```python
from build123d import *

# Parameters (mm, degrees)
ESQUISSE1_W              = 137
ESQUISSE1_H              = 66
BOSS_EXTRU_2_DEPTH       = 15
ESQUISSE3_W              = 131
ESQUISSE3_H              = 60
ENL_V_MAT_EXTRU_1_DEPTH  = 10
ESQUISSE5_W              = 12
ESQUISSE5_H              = 12
ENL_V_MAT_EXTRU_2_DEPTH  = 10
ESQUISSE6_W              = 12
ESQUISSE6_H              = 12
ENL_V_MAT_EXTRU_3_DEPTH  = 10
ESQUISSE7_W              = 15
ESQUISSE7_H              = 3
ENL_V_MAT_EXTRU_4_DEPTH  = 10
ESQUISSE8_R              = 4.5
ENL_V_MAT_EXTRU_5_DEPTH  = 10
ESQUISSE10_W             = 3
ESQUISSE10_H             = 8
BOSS_EXTRU_3_DEPTH       = 4
ESQUISSE12_W             = 2
ESQUISSE12_H             = 6
ENL_V_MAT_EXTRU_6_DEPTH  = 4
ESQUISSE13_W             = 3
ESQUISSE13_H             = 8
BOSS_EXTRU_4_DEPTH       = 4
ESQUISSE14_W             = 2
ESQUISSE14_H             = 6
ENL_V_MAT_EXTRU_7_DEPTH  = 4
ESQUISSE16_W             = 3
ESQUISSE16_H             = 8
BOSS_EXTRU_5_DEPTH       = 4
ESQUISSE17_W             = 3
ESQUISSE17_H             = 8
BOSS_EXTRU_6_DEPTH       = 4
ESQUISSE19_W             = 2
ESQUISSE19_H             = 6
ENL_V_MAT_EXTRU_9_DEPTH  = 3
ESQUISSE20_W             = 2
ESQUISSE20_H             = 6
ENL_V_MAT_EXTRU_10_DEPTH = 3
ESQUISSE21_R             = 1.5
ENL_V_MAT_EXTRU_12_DEPTH = 21
ESQUISSE22_W             = 3
ESQUISSE22_H             = 8
ENL_V_MAT_EXTRU_13_DEPTH = 4
ESQUISSE23_W             = 3
ESQUISSE23_H             = 8
ENL_V_MAT_EXTRU_14_DEPTH = 4
ESQUISSE24_W             = 3
ESQUISSE24_H             = 8
ENL_V_MAT_EXTRU_15_DEPTH = 4
ESQUISSE25_W             = 3
ESQUISSE25_H             = 8
ENL_V_MAT_EXTRU_16_DEPTH = 4
ESQUISSE28_W             = 12
ESQUISSE28_H             = 12
BOSS_EXTRU_7_DEPTH       = 5
ESQUISSE30_W             = 9
ESQUISSE30_H             = 9
ENL_V_MAT_EXTRU_17_DEPTH = 2.5
ESQUISSE32_W             = 9
ESQUISSE32_H             = 9
ENL_V_MAT_EXTRU_18_DEPTH = 8.5
ESQUISSE33_W             = 16
ESQUISSE33_H             = 16
ENL_V_MAT_EXTRU_19_DEPTH = 3
ESQUISSE34_W             = 16
ESQUISSE34_H             = 16
ENL_V_MAT_EXTRU_20_DEPTH = 3
ESQUISSE35_W             = 9
ESQUISSE35_H             = 9
ENL_V_MAT_EXTRU_21_DEPTH = 3
ESQUISSE36_W             = 12
ESQUISSE36_H             = 12
BOSS_EXTRU_8_DEPTH       = 5
ESQUISSE37_R             = 2.5
ENL_V_MAT_EXTRU_22_DEPTH = 5
ESQUISSE39_W             = 3
ESQUISSE39_H             = 60
ENL_V_MAT_EXTRU_23_DEPTH = 10
ESQUISSE40_W             = 5
ESQUISSE40_H             = 66
BOSS_EXTRU_9_DEPTH       = 7
ESQUISSE41_W             = 3
ESQUISSE41_H             = 66
BOSS_EXTRU_10_DEPTH      = 10
ESQUISSE42_W             = 4
ESQUISSE42_H             = 3
BOSS_EXTRU_11_DEPTH      = 10
ESQUISSE43_W             = 4
ESQUISSE43_H             = 3
BOSS_EXTRU_12_DEPTH      = 10
ESQUISSE44_W             = 20
ESQUISSE44_H             = 8
ENL_V_MAT_EXTRU_24_DEPTH = 10
ESQUISSE46_W             = 138
ESQUISSE46_H             = 3
ENL_V_MAT_EXTRU_25_DEPTH = 10
ESQUISSE47_W             = 141
ESQUISSE47_H             = 5
BOSS_EXTRU_13_DEPTH      = 7
ESQUISSE48_W             = 141
ESQUISSE48_H             = 3.004636282
BOSS_EXTRU_14_DEPTH      = 10
ESQUISSE49_W             = 3
ESQUISSE49_H             = 3.995363718
BOSS_EXTRU_15_DEPTH      = 10
ESQUISSE50_W             = 3
ESQUISSE50_H             = 15
BOSS_EXTRU_16_DEPTH      = 7


with BuildPart() as part:
    # Esquisse1 → Boss.-Extru.2 (new body)
    with BuildSketch(Plane.XY):
        with Locations((68.5, 33)):
            Rectangle(ESQUISSE1_W, ESQUISSE1_H)
    extrude(amount=BOSS_EXTRU_2_DEPTH)

    # Esquisse3 → Enlèv. mat.-Extru.1 (cut)
    with BuildSketch(Plane.XY.offset(15)):
        with Locations((68.5, 33)):
            Rectangle(ESQUISSE3_W, ESQUISSE3_H)
    extrude(amount=-ENL_V_MAT_EXTRU_1_DEPTH, mode=Mode.SUBTRACT)

    # Esquisse5 → Enlèv. mat.-Extru.2 (cut)
    with BuildSketch(Plane(origin=(0, 0, 0), x_dir=(-1, 0, 0), z_dir=(0, 0, -1))):
        with Locations((-14.887820014, 52.506524993)):
            Rectangle(ESQUISSE5_W, ESQUISSE5_H)
    extrude(amount=-ENL_V_MAT_EXTRU_2_DEPTH, mode=Mode.SUBTRACT)

    # Esquisse6 → Enlèv. mat.-Extru.3 (cut)
    with BuildSketch(Plane(origin=(0, 0, 0), x_dir=(-1, 0, 0), z_dir=(0, 0, -1))):
        with Locations((-42.758546676, 52.506524993)):
            Rectangle(ESQUISSE6_W, ESQUISSE6_H)
    extrude(amount=-ENL_V_MAT_EXTRU_3_DEPTH, mode=Mode.SUBTRACT)

    # Esquisse7 → Enlèv. mat.-Extru.4 (cut)
    with BuildSketch(Plane(origin=(0, 0, 0), x_dir=(-1, 0, 0), z_dir=(0, 0, -1))):
        with Locations((-55.331883335, 4.5)):
            Rectangle(ESQUISSE7_W, ESQUISSE7_H)
    extrude(amount=-ENL_V_MAT_EXTRU_4_DEPTH, mode=Mode.SUBTRACT)

    # Esquisse8 → Enlèv. mat.-Extru.5 (cut)
    with BuildSketch(Plane(origin=(0, 0, 0), x_dir=(-1, 0, 0), z_dir=(0, 0, -1))):
        with Locations((-69.128546676, 52.506524993)):
            Circle(ESQUISSE8_R)
    extrude(amount=-ENL_V_MAT_EXTRU_5_DEPTH, mode=Mode.SUBTRACT)

    # Esquisse10 → Boss.-Extru.3 (add)
    with BuildSketch(Plane.XY.offset(5)):
        with Locations((7.387820014, 52.506524993)):
            Rectangle(ESQUISSE10_W, ESQUISSE10_H)
    extrude(amount=BOSS_EXTRU_3_DEPTH)

    # Esquisse12 → Enlèv. mat.-Extru.6 (cut)
    with BuildSketch(Plane(origin=(8.887820014, 0, 0), x_dir=(0, 0, -1), z_dir=(1, 0, 0))):
        with Locations((-7, 52.506524993)):
            Rectangle(ESQUISSE12_W, ESQUISSE12_H)
    extrude(amount=-ENL_V_MAT_EXTRU_6_DEPTH, mode=Mode.SUBTRACT)

    # Esquisse13 → Boss.-Extru.4 (add)
    with BuildSketch(Plane.XY.offset(5)):
        with Locations((22.387820014, 52.506524993)):
            Rectangle(ESQUISSE13_W, ESQUISSE13_H)
    extrude(amount=BOSS_EXTRU_4_DEPTH)

    # Esquisse14 → Enlèv. mat.-Extru.7 (cut)
    with BuildSketch(Plane(origin=(23.887820014, 0, 0), x_dir=(0, 0, -1), z_dir=(1, 0, 0))):
        with Locations((-7, 52.506524993)):
            Rectangle(ESQUISSE14_W, ESQUISSE14_H)
    extrude(amount=-ENL_V_MAT_EXTRU_7_DEPTH, mode=Mode.SUBTRACT)

    # Esquisse16 → Boss.-Extru.5 (add)
    with BuildSketch(Plane.XY.offset(5)):
        with Locations((35.258546676, 52.506524993)):
            Rectangle(ESQUISSE16_W, ESQUISSE16_H)
    extrude(amount=BOSS_EXTRU_5_DEPTH)

    # Esquisse17 → Boss.-Extru.6 (add)
    with BuildSketch(Plane.XY.offset(5)):
        with Locations((50.258546676, 52.506524993)):
            Rectangle(ESQUISSE17_W, ESQUISSE17_H)
    extrude(amount=BOSS_EXTRU_6_DEPTH)

    # Esquisse19 → Enlèv. mat.-Extru.9 (cut)
    with BuildSketch(Plane(origin=(36.758546676, 0, 0), x_dir=(0, 0, -1), z_dir=(1, 0, 0))):
        with Locations((-7, 52.506524993)):
            Rectangle(ESQUISSE19_W, ESQUISSE19_H)
    extrude(amount=-ENL_V_MAT_EXTRU_9_DEPTH, mode=Mode.SUBTRACT)

    # Esquisse20 → Enlèv. mat.-Extru.10 (cut)
    with BuildSketch(Plane(origin=(51.758546676, 0, 0), x_dir=(0, 0, -1), z_dir=(1, 0, 0))):
        with Locations((-7, 52.506524993)):
            Rectangle(ESQUISSE20_W, ESQUISSE20_H)
    extrude(amount=-ENL_V_MAT_EXTRU_10_DEPTH, mode=Mode.SUBTRACT)

    # Esquisse21 → Enlèv. mat.-Extru.12 (cut)
    with BuildSketch(Plane(origin=(0, 0, 0), x_dir=(-1, 0, 0), z_dir=(0, 0, -1))):
        with Locations((-90.998546676, 52.506524993)):
            Circle(ESQUISSE21_R)
    extrude(amount=-ENL_V_MAT_EXTRU_12_DEPTH, mode=Mode.SUBTRACT)

    # Esquisse22 → Enlèv. mat.-Extru.13 (cut)
    with BuildSketch(Plane.XY.offset(9)):
        with Locations((50.258546676, 52.506524993)):
            Rectangle(ESQUISSE22_W, ESQUISSE22_H)
    extrude(amount=-ENL_V_MAT_EXTRU_13_DEPTH, mode=Mode.SUBTRACT)

    # Esquisse23 → Enlèv. mat.-Extru.14 (cut)
    with BuildSketch(Plane.XY.offset(9)):
        with Locations((35.258546676, 52.506524993)):
            Rectangle(ESQUISSE23_W, ESQUISSE23_H)
    extrude(amount=-ENL_V_MAT_EXTRU_14_DEPTH, mode=Mode.SUBTRACT)

    # Esquisse24 → Enlèv. mat.-Extru.15 (cut)
    with BuildSketch(Plane.XY.offset(9)):
        with Locations((22.387820014, 52.506524993)):
            Rectangle(ESQUISSE24_W, ESQUISSE24_H)
    extrude(amount=-ENL_V_MAT_EXTRU_15_DEPTH, mode=Mode.SUBTRACT)

    # Esquisse25 → Enlèv. mat.-Extru.16 (cut)
    with BuildSketch(Plane.XY.offset(9)):
        with Locations((7.387820014, 52.506524993)):
            Rectangle(ESQUISSE25_W, ESQUISSE25_H)
    extrude(amount=-ENL_V_MAT_EXTRU_16_DEPTH, mode=Mode.SUBTRACT)

    # Esquisse28 → Boss.-Extru.7 (add)
    with BuildSketch(Plane(origin=(0, 0, 0), x_dir=(-1, 0, 0), z_dir=(0, 0, -1))):
        with Locations((-14.887820014, 52.506524993)):
            Rectangle(ESQUISSE28_W, ESQUISSE28_H)
    extrude(amount=-BOSS_EXTRU_7_DEPTH)

    # Esquisse30 → Enlèv. mat.-Extru.17 (cut)
    with BuildSketch(Plane.XY.offset(5)):
        with Locations((23.793387087, 33.541365404)):
            Rectangle(ESQUISSE30_W, ESQUISSE30_H)
    extrude(amount=-ENL_V_MAT_EXTRU_17_DEPTH, mode=Mode.SUBTRACT)

    # Esquisse32 → Enlèv. mat.-Extru.18 (cut)
    with BuildSketch(Plane.XY.offset(5)):
        with Locations((23.793387087, 33.541365404)):
            Rectangle(ESQUISSE32_W, ESQUISSE32_H)
    extrude(amount=-ENL_V_MAT_EXTRU_18_DEPTH, mode=Mode.SUBTRACT)

    # Esquisse33 → Enlèv. mat.-Extru.19 (cut)
    with BuildSketch(Plane(origin=(0, 0, 0), x_dir=(-1, 0, 0), z_dir=(0, 0, -1))):
        with Locations((-23.76482076, 33.512799076)):
            Rectangle(ESQUISSE33_W, ESQUISSE33_H)
    extrude(amount=-ENL_V_MAT_EXTRU_19_DEPTH, mode=Mode.SUBTRACT)

    # Esquisse34 → Enlèv. mat.-Extru.20 (cut)
    with BuildSketch(Plane(origin=(0, 0, 0), x_dir=(-1, 0, 0), z_dir=(0, 0, -1))):
        with Locations((-59.43745725, 33.512799076)):
            Rectangle(ESQUISSE34_W, ESQUISSE34_H)
    extrude(amount=-ENL_V_MAT_EXTRU_20_DEPTH, mode=Mode.SUBTRACT)

    # Esquisse35 → Enlèv. mat.-Extru.21 (cut)
    with BuildSketch(Plane(origin=(0, 0, 3), x_dir=(-1, 0, 0), z_dir=(0, 0, -1))):
        with Locations((-59.688365981, 33.763707808)):
            Rectangle(ESQUISSE35_W, ESQUISSE35_H)
    extrude(amount=-ENL_V_MAT_EXTRU_21_DEPTH, mode=Mode.SUBTRACT)

    # Esquisse36 → Boss.-Extru.8 (add)
    with BuildSketch(Plane(origin=(0, 0, 0), x_dir=(-1, 0, 0), z_dir=(0, 0, -1))):
        with Locations((-42.758546676, 52.506524993)):
            Rectangle(ESQUISSE36_W, ESQUISSE36_H)
    extrude(amount=-BOSS_EXTRU_8_DEPTH)

    # Esquisse37 → Enlèv. mat.-Extru.22 (cut)
    with BuildSketch(Plane(origin=(0, 0, 0), x_dir=(-1, 0, 0), z_dir=(0, 0, -1))):
        with Locations((-90.998546676, 52.506524993)):
            Circle(ESQUISSE37_R)
    extrude(amount=-ENL_V_MAT_EXTRU_22_DEPTH, mode=Mode.SUBTRACT)

    # Esquisse39 → Enlèv. mat.-Extru.23 (cut)
    with BuildSketch(Plane.XY.offset(15)):
        with Locations((1.5, 33)):
            Rectangle(ESQUISSE39_W, ESQUISSE39_H)
    extrude(amount=-ENL_V_MAT_EXTRU_23_DEPTH, mode=Mode.SUBTRACT)

    # Esquisse40 → Boss.-Extru.9 (add)
    with BuildSketch(Plane.ZY):
        with Locations((2.5, 33)):
            Rectangle(ESQUISSE40_W, ESQUISSE40_H)
    extrude(amount=BOSS_EXTRU_9_DEPTH)

    # Esquisse41 → Boss.-Extru.10 (add)
    with BuildSketch(Plane.XY.offset(5)):
        with Locations((-5.5, 33)):
            Rectangle(ESQUISSE41_W, ESQUISSE41_H)
    extrude(amount=BOSS_EXTRU_10_DEPTH)

    # Esquisse42 → Boss.-Extru.11 (add)
    with BuildSketch(Plane.XY.offset(5)):
        with Locations((-2, 1.5)):
            Rectangle(ESQUISSE42_W, ESQUISSE42_H)
    extrude(amount=BOSS_EXTRU_11_DEPTH)

    # Esquisse43 → Boss.-Extru.12 (add)
    with BuildSketch(Plane.XY.offset(5)):
        with Locations((-2, 64.5)):
            Rectangle(ESQUISSE43_W, ESQUISSE43_H)
    extrude(amount=BOSS_EXTRU_12_DEPTH)

    # Esquisse44 → Enlèv. mat.-Extru.24 (cut)
    with BuildSketch(Plane.XY.offset(5)):
        with Locations((54.216853372, 7)):
            Rectangle(ESQUISSE44_W, ESQUISSE44_H)
    extrude(amount=-ENL_V_MAT_EXTRU_24_DEPTH, mode=Mode.SUBTRACT)

    # Esquisse46 → Enlèv. mat.-Extru.25 (cut)
    with BuildSketch(Plane.XY.offset(5)):
        with Locations((65, 64.5)):
            Rectangle(ESQUISSE46_W, ESQUISSE46_H)
    extrude(amount=ENL_V_MAT_EXTRU_25_DEPTH, mode=Mode.SUBTRACT)

    # Esquisse47 → Boss.-Extru.13 (add)
    with BuildSketch(Plane(origin=(0, 66, 0), x_dir=(1, 0, 0), z_dir=(0, 1, 0))):
        with Locations((63.5, -2.5)):
            Rectangle(ESQUISSE47_W, ESQUISSE47_H)
    extrude(amount=BOSS_EXTRU_13_DEPTH)

    # Esquisse48 → Boss.-Extru.14 (add)
    with BuildSketch(Plane.XY.offset(5)):
        with Locations((63.5, 71.497681859)):
            Rectangle(ESQUISSE48_W, ESQUISSE48_H)
    extrude(amount=BOSS_EXTRU_14_DEPTH)

    # Esquisse49 → Boss.-Extru.15 (add)
    with BuildSketch(Plane.XY.offset(5)):
        with Locations((-5.5, 67.997681859)):
            Rectangle(ESQUISSE49_W, ESQUISSE49_H)
    extrude(amount=BOSS_EXTRU_15_DEPTH)

    # Esquisse50 → Boss.-Extru.16 (add)
    with BuildSketch(Plane(origin=(0, 66, 0), x_dir=(1, 0, 0), z_dir=(0, 1, 0))):
        with Locations((135.5, -7.5)):
            Rectangle(ESQUISSE50_W, ESQUISSE50_H)
    extrude(amount=BOSS_EXTRU_16_DEPTH)


solid = part.part
```
Input: part model. Units: mm. Frame: model coordinates. A direction names the side the tool comes from. Coordinates: 2 decimals unless noted, no trailing zeros. Order: outer loops, then holes, each group sorted by start corner. A loop starts at its lowest first (then second) coordinate and runs counter-clockwise, first axis right, second up. Notation, with made-up numbers: (-25.75, 27.5) - (12.25, 27.5) arc R14 ccw to (12.25, 46.5) - close; hole circle Ø2 at (38.25, 8.25). An arc over 180 degrees is marked (long way). Return JSON: item names as keys, results as strings.
Q1. Cut plane D-D (x = 24). Return loops of the section in (y, z), then the cut area to 3 significant figures.
The answers:
{"outline": "(0, 0) - (25.51, 0) - (25.51, 3) - (29.04, 3) - (29.04, 5) - (3, 5) - (3, 15) - (0, 15) - close; (38.04, 3) - (41.51, 3) - (41.51, 0) - (73, 0) - (73, 15) - (70, 15) - (70, 5) - (38.04, 5) - close", "area": "359 mm2"}
Q2. Ray query, probe 1 along Y at (x, z) = (61, 1); probe 2 along X at (y, z) = (36, 2.75); probe 3 along Y at (x, z) = (125, 7.5). Return the intervals inside material, ascending.
The answers:
{"probe 1": "y = 0 to 3, 11 to 25.51, 41.51 to 73", "probe 2": "x = -7 to 15.76, 31.76 to 51.44, 67.44 to 137", "probe 3": "y = 0 to 3, 70 to 73"}
Q3. Cut plane C-C (z = 9). Return loops of the section in (x, y).
The answers:
{"outline": "(-7, 0) - (137, 0) - (137, 73) - (-7, 73) - close; hole (-4, 3) - (134, 3) - (134, 70) - (-4, 70) - close"}
Q4. Access query for faces 5 (the flat face through (43, 71, 15)), 6 (the flat face through (60, 41.513, 1)), 7 (the flat face through (44.217, 7, 3)), 8 (the flat face through (-4, 36, 10)). Directions: +Z, -Z, +X, -X, +Y, -Y. A direction counts if a zero-diameter tool reaches every point of the face in a straight line with its end or side. Return the directions, or none.
The answers:
{"face 5": "+Z, +X, -X, +Y, -Y", "face 6": "-Z", "face 7": "+Z, -Z", "face 8": "+Z"}
Q5. Cut plane B-B (x = 83). Return loops of the section in (y, z), then the cut area to 3 significant figures.
The answers:
{"outline": "(0, 0) - (73, 0) - (73, 15) - (70, 15) - (70, 5) - (3, 5) - (3, 15) - (0, 15) - close", "area": "425 mm2"}
Q6. Cut plane A-A (y = 31). Return loops of the section in (x, z).
The answers:
{"outline": "(-7, 0) - (15.76, 0) - (15.76, 3) - (19.29, 3) - (19.29, 5) - (-4, 5) - (-4, 15) - (-7, 15) - close; (28.29, 3) - (31.76, 3) - (31.76, 0) - (51.44, 0) - (51.44, 3) - (55.19, 3) - (55.19, 5) - (28.29, 5) - close; (64.19, 3) - (67.44, 3) - (67.44, 0) - (137, 0) - (137, 15) - (134, 15) - (134, 5) - (64.19, 5) - close"}
Q7. Draft query along Y for faces 1 (the flat face through (64, 73, 7)), 2 (the flat face through (-7, 36, 7)), 3 (the flat face through (15.765, 33, 1)), 4 (the flat face through (64, 0, 7)). Return one class per face: +Y half, -Y half, draft (parallel to the pull), parting line (faces both ways), or undercut.
The answers:
{"face 1": "+Y half", "face 2": "draft", "face 3": "undercut", "face 4": "-Y half"}
Q8. First-contact query: pin 1 (14.5 mm diameter, centred on x = 69.13, y = 52.51, fed in from +Z). Flat tip, straight axial feed; report the tip coordinate or a pass-through.
The answers:
{"pin 1": "stops at z = 5"}
